Geometry check sheet. Reference: the model listing, model coordinates, mm. Coordinates: 2 decimals unless noted, no trailing zeros. Order: outer loops, then holes, each group sorted by start corner. A loop starts at its lowest first (then second) coordinate and runs counter-clockwise, first axis right, second up. Notation, with made-up numbers: (41.5, -8) - (65.5, -8) arc R6 ccw to (65.5, 2) - close; hole circle Ø9 at (-32.5, -15.75). An arc over 180 degrees is marked (long way). Return JSON: item names as keys, results as strings. Group by question number.
Item 1: Section check C-C on y = -0.15. Enter the section's corners in (x, z) (1 decimal), then the cut area to 3 significant figures.
Item 2: Scan lines: probe 1 along Z at (x, y) = (0, -0.1); probe 2 along X at (y, z) = (-0.2, 0.25); probe 3 along Z at (x, y) = (7, -0.15). Record each from-to range of solid material in increasing order.
Item 3: Section check B-B on z = 0. Enter the section's corners in (x, y).
Item 4: Section check D-D on z = 11.43. Enter the section's corners in (x, y).
Item 5: Gauge pin test, flat ends, axial feed: pin 1 (10 mm diameter, centred on x = -1, z = -7.5, fed in from +Y); pin 2 (1.7 mm diameter, centred on x = 0, z = 11.43, fed in from +Y). Record the tip position at first contact, or that the pin passes through.
Item 6: Section check A-A on x = 0. Enter the section's corners in (y, z).
from build123d import *

# Parameters (mm, degrees)
F0_R     = 12.7
F0_R_2   = 7.62
F1_DEPTH = 0.254
F2_R     = 0.9525
F3_DEPTH = 25.4


with BuildPart() as f1:
    # F0 (on Front) → F1 (new body)
    with BuildSketch(Plane.XZ):
        Circle(F0_R)
        Circle(F0_R_2, mode=Mode.SUBTRACT)
    extrude(amount=F1_DEPTH)

    # F2 (on face) → F3 (cut)
    with BuildSketch(Plane.XZ.offset(0.254)):
        with Locations((0, 11.43)):
            Circle(F2_R)
        with Locations((11.43, 0)):
            Circle(F2_R)
        with Locations((0, -11.43)):
            Circle(F2_R)
        with Locations((-11.43, 0)):
            Circle(F2_R)
    extrude(amount=-F3_DEPTH, mode=Mode.SUBTRACT)


solid = f1.part
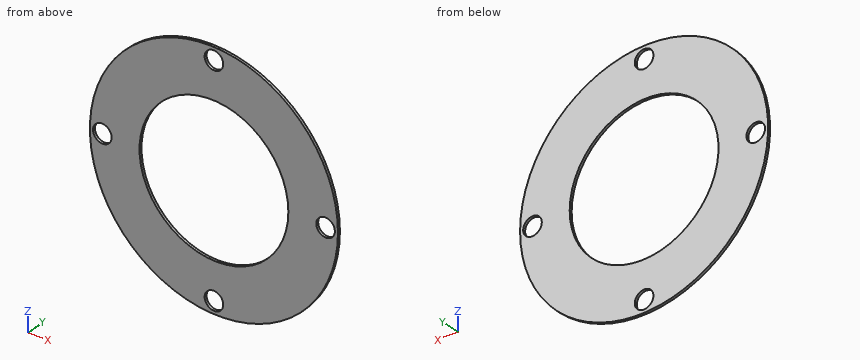
Computed:
{
 "1": {"outline": "circle Ø25.4 at (0, 0); hole circle Ø1.9 at (-11.4, 0); hole circle Ø15.2 at (0, 0); hole circle Ø1.9 at (0, -11.4); hole circle Ø1.9 at (0, 11.4); hole circle Ø1.9 at (11.4, 0)", "area": "313 mm²"},
 "2": {"probe 1": "z = -12.7 to -12.38, -10.48 to -7.62, 7.62 to 10.48, 12.38 to 12.7", "probe 2": "x = -12.7 to -12.35, -10.51 to -7.62, 7.62 to 10.51, 12.35 to 12.7", "probe 3": "z = -10.6 to -3.01, 3.01 to 10.6"},
 "3": {"outline": "(-12.7, -0.25) - (-12.38, -0.25) - (-12.38, 0) - (-12.7, 0) - close; (-10.48, -0.25) - (-7.62, -0.25) - (-7.62, 0) - (-10.48, 0) - close; (7.62, -0.25) - (10.48, -0.25) - (10.48, 0) - (7.62, 0) - close; (12.38, -0.25) - (12.7, -0.25) - (12.7, 0) - (12.38, 0) - close"},
 "4": {"outline": "(-5.54, -0.25) - (-0.95, -0.25) - (-0.95, 0) - (-5.54, 0) - close; (0.95, -0.25) - (5.54, -0.25) - (5.54, 0) - (0.95, 0) - close"},
 "5": {"pin 1": "stops at y = 0", "pin 2": "passes through"},
 "6": {"outline": "(-0.25, -12.7) - (0, -12.7) - (0, -12.38) - (-0.25, -12.38) - close; (-0.25, -10.48) - (0, -10.48) - (0, -7.62) - (-0.25, -7.62) - close; (-0.25, 7.62) - (0, 7.62) - (0, 10.48) - (-0.25, 10.48) - close; (-0.25, 12.38) - (0, 12.38) - (0, 12.7) - (-0.25, 12.7) - close"}
}
